from build123d import *

# Parameters (mm, degrees)
F3_D     = 9.525
F3_DEPTH = 9.525
F3_TIP   = 2.8615986981
F5_D     = 3.175
F5_DEPTH = 21.844
F5_TIP   = 0.9538662327


with BuildPart() as f1:
    # F0 (on Front) → F1 (revolve)
    with BuildSketch(Plane.XZ):
        with BuildLine():
            Line((-2.54, -28.544438532), (0, -28.544438532))
            Line((0, -28.544438532), (0, 0))
            Line((0, 0), (-28.575, 0))
            add(Edge.make_bspline(
                [(-28.575, 0), (-22.1033814669, -1.3008907493), (-6.7932074564, -2.9181800603), (-4.8525862527, -21.5668183457), (-2.54, -28.544438532)],
                knots=[0, 0, 0, 0, 0.476190706, 1, 1, 1, 1], degree=3))
        make_face()
        Polygon((-28.575, 0), (0, 0), (0, 9.555561468), (-10.16, 9.555561468), align=None)
    revolve(axis=Axis((0, 0, -9.494438532), (0, 0, 1)))

    # F3
    with Locations(Plane.XY.offset(9.555561468)):
        with Locations((0, 0)):
            Hole(F3_D / 2, depth=F3_DEPTH)
            with Locations((0, 0, -(F3_DEPTH + F3_TIP / 2))):  # 118° drill point
                Cone(0, F3_D / 2, F3_TIP, mode=Mode.SUBTRACT)

    # F5
    with Locations(Plane(origin=(0, 0, -28.544438532), x_dir=(1, 0, 0), z_dir=(0, 0, -1))):
        with Locations((0, 0)):
            Hole(F5_D / 2, depth=F5_DEPTH)
            with Locations((0, 0, -(F5_DEPTH + F5_TIP / 2))):  # 118° drill point
                Cone(0, F5_D / 2, F5_TIP, mode=Mode.SUBTRACT)


solid = f1.part
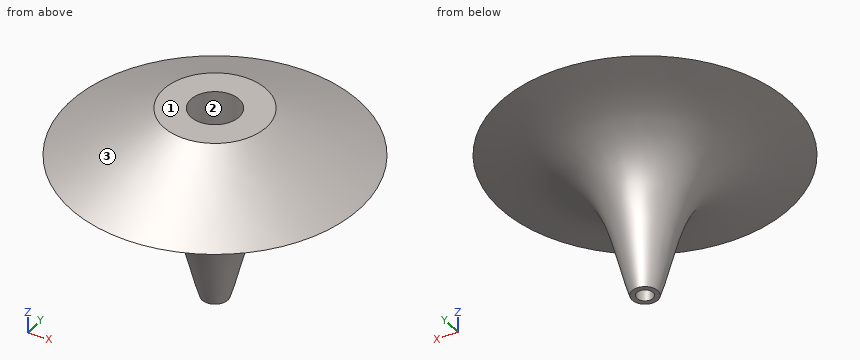
The model under review builds one solid part; all positions refer to its coordinate system, in mm. Face numbers are marked on the shaded views. Give positions to 0.01 mm unless a question says otherwise; leave off trailing zeros. Write each loop counter-clockwise with the first axis right and the second up, starting at its lowest first coordinate (ties: lowest second). Pieces come first, ordered by that corner, then holes. Notation, with made-up numbers: M -39,-16.5 L 1,-16.5 A24 ccw 1,-6.5 Z; hole C -25,-28 d3. An arc over 180 degrees is marked long. One line per question, with ' | ' between items. Start each with the question number.
Item 1: Wall thickness on line 1 (Y direction, x = 0, z = -16); line 2 (Y direction, x = 0, z = 4.5); line 3 (X direction, y = 0, z = 7): over which ranges is each line inside the solid? List them lowest first. Write a range as from..to.
Item 2: Draft analysis for pull direction X (two halves, no side actions). For the marked faces 1, 2 and 3, state which applies: released by +X, released by -X, zero draft, split by the parting line, or undercut.
Item 3: For pin 1 (1 mm diameter, centred on x = 8.5, y = 6, fed in from -Z); pin 2 (1 mm diameter, centred on x = -20, y = 14.5, fed in from -Z); pin 3 (2 mm diameter, centred on y = -12, z = 4, fed in from +X), all flat-tipped, find the tip position at first contact; note any pin that passes through.
Item 4: We need section A-A on z = 4.5. Write out the cut boundary in (x, y) (1 decimal), plus the area to 3 significant figures.
Results found:
1) line 1: y = -5.93..-1.59, 1.59..5.93 | line 2: y = -19.9..-4.76, 4.76..19.9 | line 3: x = -15.08..-4.76, 4.76..15.08
2) face 1: zero draft | face 2: undercut | face 3: split by the parting line
3) pin 1: stops at z = -7.47 | pin 2: stops at z = -0.83 | pin 3: stops at x = 19.46
4) outline: C 0,0 d39.8; hole C 0,0 d9.5 | area: 1,170 mm2
